```python
from build123d import *

# Parameters (mm, degrees)
SKETCH1_W           = 3
SKETCH1_H           = 20
SKETCH1_W_2         = 72
SKETCH1_R           = 3
BOSS_EXTRUDE2_DEPTH = 3
SKETCH1_3_W         = 3
SKETCH1_3_H         = 20
BOSS_EXTRUDE3_DEPTH = 23


with BuildPart() as part:
    # Sketch1 → Boss-Extrude2 (new body)
    with BuildSketch(Plane.XY):
        with Locations((1.5, 10)):
            Rectangle(SKETCH1_W, SKETCH1_H)
        with Locations((39, 10)):
            Rectangle(SKETCH1_W_2, SKETCH1_H)
        with Locations((20, 10)):
            Circle(SKETCH1_R, mode=Mode.SUBTRACT)
        with Locations((60, 10)):
            Circle(SKETCH1_R, mode=Mode.SUBTRACT)
    extrude(amount=BOSS_EXTRUDE2_DEPTH)

    # Sketch1_3 → Boss-Extrude3 (add)
    with BuildSketch(Plane.XY):
        with Locations((1.5, 10)):
            Rectangle(SKETCH1_3_W, SKETCH1_3_H)
    extrude(amount=-BOSS_EXTRUDE3_DEPTH)


solid = part.part
```
CAD build for the part. Positions are in the model's coordinates, mm. A direction names the side the tool comes from. Coordinates: 2 decimals unless noted, no trailing zeros. Write each loop counter-clockwise with the first axis right and the second up, starting at its lowest first coordinate (ties: lowest second). Pieces come first, ordered by that corner, then holes.
(1) Two-plate mould, pull along Y, no slides. Class faces 1 (the face through (37, 10, 3)), 2 (the face through (29, 20, 1)), 3 (the face through (17, 10, 1)): +Y half, -Y half, draft (parallel to the pull), parting line (faces both ways), or undercut.
(2) 3-axis set-ups, long thin cutter, end or side, ignore diameter. For faces 4 (the face through (57, 10, 1)), 5 (the face through (3, 10, -11)): which of +Z, -Z, +X, -X, +Y, -Y reach the whole face in a straight line?
(3) Drill centre lines: probe 1 along Y at (x, z) = (60, 2.15); probe 2 along Z at (x, y) = (8, 4). Where is each one in solid material? Low to high.
(4) Cut at C-C, the plane y = 17.75. List the corners of the cut face in (x, z).
(5) Flat gauge pin, fed straight in: pin 1 (7 mm diameter, centred on x = 20, y = 10, fed in from -Z). Where does the tip first touch, or does it go through?
(6) Cut at A-A, the plane y = 10. List the corners of the cut face in (x, z).
(7) Cut at B-B, the plane x = 20. List the corners of the cut face in (y, z).
(8) Cut at D-D, the plane z = -20.5. List the corners of the cut face in (x, y), and give its area (3 significant figures).
Geometry says:
1. face 1: draft
1. face 2: +Y half
1. face 3: undercut
2. face 4: +Z, -Z
2. face 5: -Z, +X, +Y, -Y
3. probe 1: y = 0 to 7, 13 to 20
3. probe 2: z = 0 to 3
4. outline: (0, -23) - (3, -23) - (3, 0) - (75, 0) - (75, 3) - (0, 3) - close
5. pin 1: stops at z = 0
6. outline: (0, -23) - (3, -23) - (3, 0) - (17, 0) - (17, 3) - (0, 3) - close; (23, 0) - (57, 0) - (57, 3) - (23, 3) - close; (63, 0) - (75, 0) - (75, 3) - (63, 3) - close
7. outline: (0, 0) - (7, 0) - (7, 3) - (0, 3) - close; (13, 0) - (20, 0) - (20, 3) - (13, 3) - close
8. outline: (0, 0) - (3, 0) - (3, 20) - (0, 20) - close
8. area: 60.0 mm2
